The listing builds one solid part. Answer for the finished solid, in the listing's coordinates (mm). Give positions to 0.01 mm unless a question says otherwise; leave off trailing zeros. Loops run counter-clockwise (first coordinate to the right, second up) from the corner with the lowest first, then second, coordinate; pieces in that order, holes last. Notation, with made-up numbers: (-36.5, -15) - (-15.5, -15) arc R14 ccw to (-15.5, -9) - close; hole circle Ø3 at (49, -38). An arc over 180 degrees is marked (long way). Write item = value, one per line. Start each with the question number.
1) Consider probe 1 along Z at (x, y) = (-43.75, -1.85); probe 2 along X at (y, z) = (-0.4, 32); probe 3 along X at (y, z) = (-1.7, 31.5). Determine where each line is inside the solid, lowest interval first.
2) The part is cut by section A-A on y = -0.4. Write down the section's boundary in (x, z).
3) Flat-ended cylindrical pins translate along their axes: P1, Ø5.5, axis at x = -43.75, z = 31.5, coming from the +Y side; P2, Ø4.5, axis at x = -43.75, z = -31.5, coming from the +Y side. Find the tip coordinate at first contact, or state that the pin passes through.
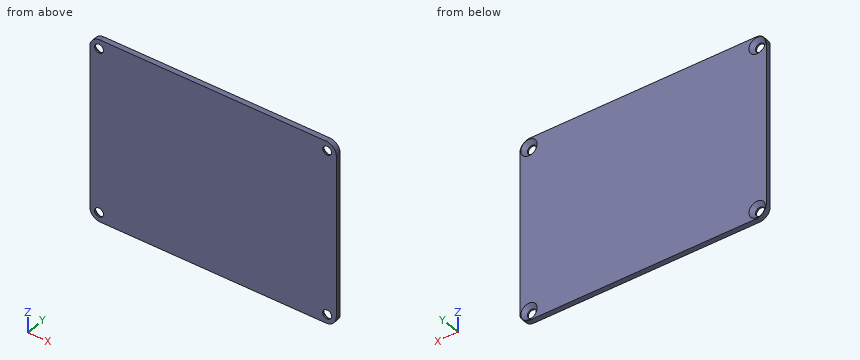
from build123d import *

# Parameters (mm, degrees)
SKETCH1_W                                       = 94.5
SKETCH1_H                                       = 70
BOSS_EXTRUDE1_DEPTH                             = 2
CSK_FOR_M3_FLAT_HEAD_MACHINE_SCREW1_D           = 3.4
CSK_FOR_M3_FLAT_HEAD_MACHINE_SCREW1_DEPTH       = 30
CSK_FOR_M3_FLAT_HEAD_MACHINE_SCREW1_CSINK_D     = 6.3
CSK_FOR_M3_FLAT_HEAD_MACHINE_SCREW1_CSINK_ANGLE = 90
CSK_FOR_M3_FLAT_HEAD_MACHINE_SCREW1_TIP         = 1.021463052
FILLET1_R                                       = 4


with BuildPart() as part:
    # Sketch1 → Boss-Extrude1 (new body)
    with BuildSketch(Plane(origin=(0, 0, 0), x_dir=(1, 0, 0), z_dir=(0, 1, 0))):
        Rectangle(SKETCH1_W, SKETCH1_H)
    extrude(amount=-BOSS_EXTRUDE1_DEPTH)

    # CSK for M3 Flat Head Machine Screw1
    with Locations(Plane(origin=(-43.75, 0, -31.5), x_dir=(0, 0, 1), z_dir=(0, 1, 0))):
        with Locations((0, 0), (0, 87.5), (63, 87.5), (63, 0)):
            CounterSinkHole(CSK_FOR_M3_FLAT_HEAD_MACHINE_SCREW1_D / 2, CSK_FOR_M3_FLAT_HEAD_MACHINE_SCREW1_CSINK_D / 2, depth=CSK_FOR_M3_FLAT_HEAD_MACHINE_SCREW1_DEPTH, counter_sink_angle=CSK_FOR_M3_FLAT_HEAD_MACHINE_SCREW1_CSINK_ANGLE)
            with Locations((0, 0, -(CSK_FOR_M3_FLAT_HEAD_MACHINE_SCREW1_DEPTH + CSK_FOR_M3_FLAT_HEAD_MACHINE_SCREW1_TIP / 2))):  # 118° drill point
                Cone(0, CSK_FOR_M3_FLAT_HEAD_MACHINE_SCREW1_D / 2, CSK_FOR_M3_FLAT_HEAD_MACHINE_SCREW1_TIP, mode=Mode.SUBTRACT)

    # Fillet1
    fillet1_edges = [part.edges().sort_by_distance(p)[0] for p in [
        (47.25, -1, 35),
        (-47.25, -1, 35),
        (-47.25, -1, -35),
        (47.25, -1, -35),
    ]]
    fillet(fillet1_edges, radius=FILLET1_R)


solid = part.part
Answer below:
q1.probe_1 = -34.97 to -33.2, -29.8 to 29.8, 33.2 to 34.97
q1.probe_2 = -47.12 to -46.45, -41.05 to 41.05, 46.45 to 47.12
q1.probe_3 = -47.22 to -45.45, -42.05 to 42.05, 45.45 to 47.22
q2.outline = (-47.25, -31) arc R4 ccw to (-43.25, -35) - (43.25, -35) arc R4 ccw to (47.25, -31) - (47.25, 31) arc R4 ccw to (43.25, 35) - (-43.25, 35) arc R4 ccw to (-47.25, 31) - close; hole circle Ø5.5 at (-43.75, -31.5); hole circle Ø5.5 at (-43.75, 31.5); hole circle Ø5.5 at (43.75, -31.5); hole circle Ø5.5 at (43.75, 31.5)
q3.P1 = -0.4
q3.P2 = -0.9
